Could you check a few things on this model? Use its own coordinates, in mm. Face numbers are marked on the shaded views. A direction names the side the tool comes from. Round coordinates to 2 decimals unless told otherwise and drop trailing zeros. Write each loop counter-clockwise with the first axis right and the second up, starting at its lowest first coordinate (ties: lowest second). Pieces come first, ordered by that corner, then holes. Notation, with made-up numbers: (-13, -39.75) -> (18, -39.75) arc R17 cw to (18, -15.75) -> close; hole circle Ø4 at (60, 32.25). An arc over 180 degrees is marked (long way). Return JSON: item names as keys, results as strings.
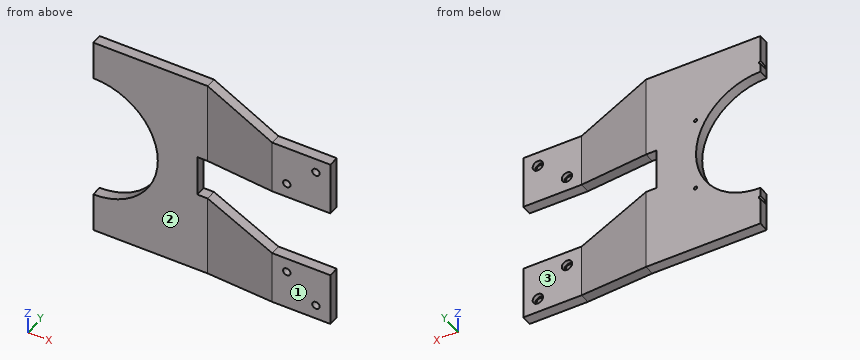
from build123d import *

# Parameters (mm, degrees)
SKETCH_1_W          = 28
SKETCH_1_H          = 26
EXTRUDE_1_DEPTH     = 5
EXTRUDE_1_2_DEPTH   = 5
EXTRUDE_START       = 10
SKETCH_1_12_W       = 50
SKETCH_1_12_H       = 100
EXTRUDE_2_DEPTH     = 5
SKETCH_2_W          = 40
SKETCH_2_H          = 5
EXTRUDE_3_DEPTH     = 5
SKETCH_3_R          = 1.8
CUT_EXTRUDE_1_DEPTH = 131.38404815
SKETCH_3_3_R        = 2.5
CUT_EXTRUDE_2_DEPTH = 2
SKETCH_4_R          = 0.75
CUT_EXTRUDE_3_DEPTH = 4
SKETCH_5_R          = 31
CUT_EXTRUDE_4_DEPTH = 131.862523333


with BuildPart() as part:
    # 草图1 → 凸台-拉伸1 (new body)
    with BuildSketch(Plane(origin=(0, 0, 0), x_dir=(1, 0, 0), z_dir=(0, 1, 0))):
        with Locations((106, 29.5)):
            Rectangle(SKETCH_1_W, SKETCH_1_H)
    extrude(amount=EXTRUDE_1_DEPTH)


with BuildPart() as body_2:
    # 草图1 → Extrude 1 2 (new body)
    with BuildSketch(Plane(origin=(0, 0, 0), x_dir=(1, 0, 0), z_dir=(0, 1, 0))):
        with Locations((106, -29.5)):
            Rectangle(SKETCH_1_W, SKETCH_1_H)
    extrude(amount=EXTRUDE_1_2_DEPTH)


with BuildPart() as body_3:
    # 草图1<12> → 凸台-拉伸2 (new body)
    with BuildSketch(Plane(origin=(0, 0, 0), x_dir=(1, 0, 0), z_dir=(0, 1, 0)).offset(EXTRUDE_START)):
        with Locations((25, 0)):
            Rectangle(SKETCH_1_12_W, SKETCH_1_12_H)
    extrude(amount=EXTRUDE_2_DEPTH)

    # 草图2 → 凸台-拉伸3 (add)
    with BuildSketch(Plane(origin=(50, 0, 0), x_dir=(0, 0, -1), z_dir=(1, 0, 0))):
        with Locations((30, 12.5)):
            Rectangle(SKETCH_2_W, SKETCH_2_H)
        with Locations((-30, 12.5)):
            Rectangle(SKETCH_2_W, SKETCH_2_H)
    extrude(amount=EXTRUDE_3_DEPTH)


    add(body_2.part)  # loft_5 joins it to this body
    # loft from a face of the part (loft_5)
    loft([body_3.faces().sort_by_distance((55, 12.5, 30))[0], body_3.faces().sort_by_distance((92, 2.5, 29.5))[0]])


    add(part.part)  # loft_6 joins it to this body
    # loft from a face of the part (loft_6)
    loft([body_3.faces().sort_by_distance((55, 12.5, -30))[0], body_3.faces().sort_by_distance((92, 2.5, -29.5))[0]])

    # 草图3 → 切除-拉伸1 (cut, through all)
    with BuildSketch(Plane(origin=(0, 5, 0), x_dir=(1, 0, 0), z_dir=(0, 1, 0))):
        with Locations(Location((113, 35.5, 0), (0, 0, 270))):
            Circle(SKETCH_3_R)
        with Locations(Location((99, 23.5, 0), (0, 0, 270))):
            Circle(SKETCH_3_R)
        with Locations(Location((113, -35.5, 0), (0, 0, 270))):
            Circle(SKETCH_3_R)
        with Locations(Location((99, -23.5, 0), (0, 0, 270))):
            Circle(SKETCH_3_R)
    extrude(amount=-CUT_EXTRUDE_1_DEPTH, mode=Mode.SUBTRACT)

    # 草图3<3> → 切除-拉伸2 (cut)
    with BuildSketch(Plane(origin=(0, 5, 0), x_dir=(1, 0, 0), z_dir=(0, 1, 0))):
        with Locations(Location((99, 23.5, 0), (0, 0, 270))):
            Circle(SKETCH_3_3_R)
        with Locations(Location((113, 35.5, 0), (0, 0, 270))):
            Circle(SKETCH_3_3_R)
        with Locations(Location((113, -35.5, 0), (0, 0, 270))):
            Circle(SKETCH_3_3_R)
        with Locations(Location((99, -23.5, 0), (0, 0, 270))):
            Circle(SKETCH_3_3_R)
    extrude(amount=-CUT_EXTRUDE_2_DEPTH, mode=Mode.SUBTRACT)

    # 草图4 → 切除-拉伸3 (cut)
    with BuildSketch(Plane(origin=(0, 15, 0), x_dir=(1, 0, 0), z_dir=(0, 1, 0))):
        with Locations((0, 36)):
            Circle(SKETCH_4_R)
        with Locations(Location((31.176914536, 18, 0), (0, 0, 270))):
            Circle(SKETCH_4_R)
        with Locations(Location((31.176914536, -18, 0), (0, 0, 270))):
            Circle(SKETCH_4_R)
        with Locations((0, -36)):
            Circle(SKETCH_4_R)
    extrude(amount=-CUT_EXTRUDE_3_DEPTH, mode=Mode.SUBTRACT)

    # 草图5 → 切除-拉伸4 (cut, through all)
    with BuildSketch(Plane(origin=(0, 15, 0), x_dir=(1, 0, 0), z_dir=(0, 1, 0))):
        Circle(SKETCH_5_R)
    extrude(amount=-CUT_EXTRUDE_4_DEPTH, mode=Mode.SUBTRACT)


solid = body_3.part
1) I want a section at B-B, the plane z = 6.5. Please give me the cut outline in (x, y).
Return value:
{"outline": "(30.31, 10) -> (50, 10) -> (50, 15) -> (30.31, 15) -> close"}
2) For the marked faces 1, 2 and 3, which set-ups out of +Z, -Z, +X, -X, +Y, -Y let a thin tool reach every point of the face, with its end or its side?
Return value:
{"face 1": "+Z, -Z, +X, -X, -Y", "face 2": "+Z, -Z, -X, -Y", "face 3": "+Z, -Z, +X, +Y"}
3) If I drill on probe 1 along Z at (x, y) = (99, 1.2); probe 2 along Y at (x, z) = (106.5, -23); probe 3 along Z at (x, y) = (73, 6.5), over which ranges is the centre line in solid material (lowest first)? Write a range as [from, to].
Return value:
{"probe 1": "[-42.5, -25.3], [-21.7, -16.5], [16.5, 21.7], [25.3, 42.5]", "probe 2": "[0, 5]", "probe 3": "[-46.35, -13.16], [13.16, 46.35]"}
4) Will these pins go through, and if not, where does the flat tip stop? pin 1 Ø4.5 at (x, z) = (113, -35.5) entering from -Y; pin 2 Ø13 at (x, z) = (113, 35) entering from +Y; pin 3 Ø1.2 at (x, z) = (31.18, -18) entering from -Y; pin 4 Ø1.5 at (x, y) = (99, 3.5) entering from +Z.
Return value:
{"pin 1": "y = 0", "pin 2": "y = 5", "pin 3": "y = 10", "pin 4": "z = 42.5"}
5) I want a section at A-A, the plane x = 113. Please give me the cut outline in (y, z), and give its area (3 significant figures).
Return value:
{"outline": "(0, -42.5) -> (5, -42.5) -> (5, -38) -> (3, -38) -> (3, -37.3) -> (0, -37.3) -> close; (0, -33.7) -> (3, -33.7) -> (3, -33) -> (5, -33) -> (5, -16.5) -> (0, -16.5) -> close; (0, 16.5) -> (5, 16.5) -> (5, 33) -> (3, 33) -> (3, 33.7) -> (0, 33.7) -> close; (0, 37.3) -> (3, 37.3) -> (3, 38) -> (5, 38) -> (5, 42.5) -> (0, 42.5) -> close", "area": "218 mm²"}
